Input: part model. Units: mm. Frame: model coordinates. Face numbers are marked on the shaded views. A direction names the side the tool comes from. Give positions to 0.01 mm unless a question says otherwise; leave off trailing zeros. Loops run counter-clockwise (first coordinate to the right, second up) from the corner with the lowest first, then second, coordinate; pieces in that order, holes last.
from build123d import *

# Parameters (mm, degrees)
SKETCH1_R               = 100
SKETCH1_R_2             = 70
BOSS_EXTRUDE1_DEPTH     = 2.5
SKETCH2_R               = 72.5
SKETCH2_R_2             = 70
BOSS_EXTRUDE2_DEPTH     = 30
SKETCH3_R               = 72.5
BOSS_EXTRUDE3_DEPTH     = 2.5
BOSS_EXTRUDE4_DEPTH     = 5
CUT_EXTRUDE1_DEPTH      = 5
CUT_EXTRUDE1_DEPTH_BACK = 146.107718609
SKETCH4_R               = 2


with BuildPart() as part:
    # Sketch1 → Boss-Extrude1 (new body)
    with BuildSketch(Plane(origin=(0, 0, 0), x_dir=(1, 0, 0), z_dir=(0, 1, 0))):
        with Locations(Location((0, 0, 0), (0, 0, 270))):
            Circle(SKETCH1_R)
        with Locations(Location((0, 0, 0), (0, 0, 270))):
            Circle(SKETCH1_R_2, mode=Mode.SUBTRACT)
    extrude(amount=BOSS_EXTRUDE1_DEPTH)

    # Sketch2 → Boss-Extrude2 (add)
    with BuildSketch(Plane(origin=(0, 2.5, 0), x_dir=(1, 0, 0), z_dir=(0, 1, 0))):
        with Locations(Location((0, 0, 0), (0, 0, 270))):
            Circle(SKETCH2_R)
        with Locations(Location((0, 0, 0), (0, 0, 270))):
            Circle(SKETCH2_R_2, mode=Mode.SUBTRACT)
    extrude(amount=BOSS_EXTRUDE2_DEPTH)

    # Sketch3 → Boss-Extrude3 (add)
    with BuildSketch(Plane(origin=(0, 32.5, 0), x_dir=(1, 0, 0), z_dir=(0, 1, 0))):
        with Locations(Location((0, 0, 0), (0, 0, 270))):
            Circle(SKETCH3_R)
    extrude(amount=BOSS_EXTRUDE3_DEPTH)

    # Sketch5 → Boss-Extrude4 (add)
    with BuildSketch(Plane.XZ):
        with BuildLine():
            ThreePointArc((69.285714286, -9.974457174), (69.821200219, -5), (70, 0))
            ThreePointArc((70, 0), (69.821200219, 5), (69.285714286, 9.974457174))
            ThreePointArc((69.285714286, 9.974457174), (60, 0), (69.285714286, -9.974457174))
        make_face()
        with BuildLine():
            ThreePointArc((26.004723841, 64.990417278), (30, 51.961524227), (43.280990445, 55.015960104))
            ThreePointArc((43.280990445, 55.015960104), (35, 60.621778265), (26.004723841, 64.990417278))
        make_face()
        with BuildLine():
            ThreePointArc((-43.280990445, 55.015960104), (-30, 51.961524227), (-26.004723841, 64.990417278))
            ThreePointArc((-26.004723841, 64.990417278), (-35, 60.621778265), (-43.280990445, 55.015960104))
        make_face()
        with BuildLine():
            ThreePointArc((-69.285714286, -9.974457174), (-60, 0), (-69.285714286, 9.974457174))
            ThreePointArc((-69.285714286, 9.974457174), (-70, 0), (-69.285714286, -9.974457174))
        make_face()
        with BuildLine():
            ThreePointArc((-43.280990445, -55.015960104), (-35, -60.621778265), (-26.004723841, -64.990417278))
            ThreePointArc((-26.004723841, -64.990417278), (-30, -51.961524227), (-43.280990445, -55.015960104))
        make_face()
        with BuildLine():
            ThreePointArc((26.004723841, -64.990417278), (35, -60.621778265), (43.280990445, -55.015960104))
            ThreePointArc((43.280990445, -55.015960104), (30, -51.961524227), (26.004723841, -64.990417278))
        make_face()
    extrude(amount=-BOSS_EXTRUDE4_DEPTH)

    # Sketch4 → Cut-Extrude1 (cut, two sides: drawn at the far end of the back side and taken through both)
    with BuildSketch(Plane(origin=(0, 2.5, 0), x_dir=(1, 0, 0), z_dir=(0, 1, 0)).offset(-CUT_EXTRUDE1_DEPTH_BACK)):
        with Locations(Location((85, 0, 0), (0, 0, 270))):
            Circle(SKETCH4_R)
        with Locations(Location((65, 0, 0), (0, 0, 270))):
            Circle(SKETCH4_R)
        with Locations(Location((32.5, -56.291651246, 0), (0, 0, 270))):
            Circle(SKETCH4_R)
        with Locations(Location((42.5, -73.612159322, 0), (0, 0, 270))):
            Circle(SKETCH4_R)
        with Locations(Location((-32.5, -56.291651246, 0), (0, 0, 270))):
            Circle(SKETCH4_R)
        with Locations(Location((-42.5, -73.612159322, 0), (0, 0, 270))):
            Circle(SKETCH4_R)
        with Locations(Location((-65, 0, 0), (0, 0, 270))):
            Circle(SKETCH4_R)
        with Locations(Location((-85, 0, 0), (0, 0, 270))):
            Circle(SKETCH4_R)
        with Locations(Location((-32.5, 56.291651246, 0), (0, 0, 270))):
            Circle(SKETCH4_R)
        with Locations(Location((-42.5, 73.612159322, 0), (0, 0, 270))):
            Circle(SKETCH4_R)
        with Locations(Location((32.5, 56.291651246, 0), (0, 0, 270))):
            Circle(SKETCH4_R)
        with Locations(Location((42.5, 73.612159322, 0), (0, 0, 270))):
            Circle(SKETCH4_R)
    extrude(amount=CUT_EXTRUDE1_DEPTH + CUT_EXTRUDE1_DEPTH_BACK, mode=Mode.SUBTRACT)


solid = part.part
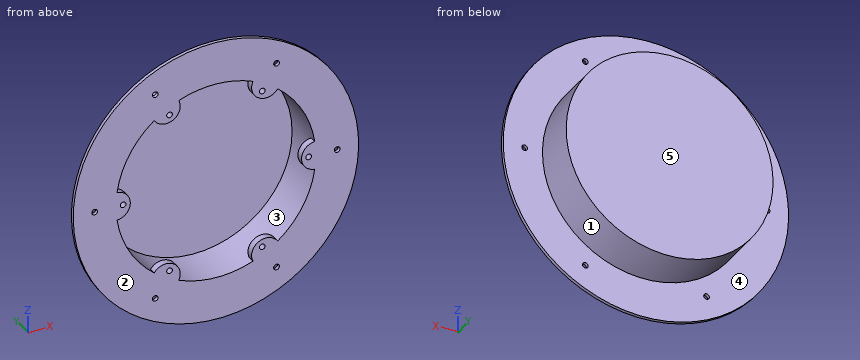
(1) Reachability of the marked faces 4 and 5 from +Z, -Z, +X, -X, +Y, -Y: full face, straight path, thin tool, end or side. Return the list, or none.
Values follow:
face 4: +Y
face 5: +Z, -Z, +X, -X, +Y
(2) Cut plane A-A (x = 0). Return the cut outline in (y, z), and give its area (4 significant figures).
Values follow:
outline: (0, -100) - (2.5, -100) - (2.5, -72.5) - (35, -72.5) - (35, 72.5) - (2.5, 72.5) - (2.5, 100) - (0, 100) - (0, 70) - (32.5, 70) - (32.5, -70) - (0, -70) - close
area: 662.5 mm2
(3) Cut plane B-B (y = 25). Return the cut outline in (x, z), and give its area (3 significant figures).
Values follow:
outline: circle Ø145 at (0, 0); hole circle Ø140 at (0, 0)
area: 1,120 mm2
(4) Pin query (flat end, axial travel): pin 1 Ø12 at (x, y) = (62, 14) entering from +Z; pin 2 Ø8 at (y, z) = (4, -74) entering from -X; pin 3 Ø5 at (x, z) = (-32.5, -56.29) entering from -Y; pin 4 Ø5 at (x, z) = (-42.5, 73.61) entering from +Y. Return the tip coordinate at first contact, or that it passes through.
Values follow:
pin 1: stops at z = 46.05
pin 2: stops at x = -71.13
pin 3: stops at y = 0
pin 4: stops at y = 2.5
(5) Cut plane C-C (z = 37). Return the cut outline in (x, y).
Values follow:
outline: (-92.9, 0) - (-59.42, 0) - (-59.42, 32.5) - (59.42, 32.5) - (59.42, 0) - (92.9, 0) - (92.9, 2.5) - (62.35, 2.5) - (62.35, 35) - (-62.35, 35) - (-62.35, 2.5) - (-92.9, 2.5) - close
(6) Mould query, pull axis X, two halves, no side actions, for the marked faces 1, 2 and 3. Classes: +X half, -X half, draft (parallel to the pull), parting line (faces both ways), or undercut.
Values follow:
face 1: parting line
face 2: draft
face 3: undercut
(7) Ray query, probe 1 along Z at (x, y) = (32.5, 1.4); probe 2 along X at (y, z) = (22, 2); probe 3 along Y at (x, z) = (29, 7). Return the intervals inside material, ascending.
Values follow:
probe 1: z = -94.57 to -58.29, -54.29 to -50.94, 50.94 to 54.29, 58.29 to 94.57
probe 2: x = -72.47 to -69.97, 69.97 to 72.47
probe 3: y = 32.5 to 35
